Model file for the job. Use its own axes, mm. Face numbers are marked on the shaded views. A direction names the side the tool comes from. Coordinates: 2 decimals unless noted, no trailing zeros. Order: outer loops, then holes, each group sorted by start corner. A loop starts at its lowest first (then second) coordinate and runs counter-clockwise, first axis right, second up. Notation, with made-up numbers: M -1,33.25 L 27,33.25 A27 ccw 27,65.25 Z; hole C 23,65.5 d5. An arc over 180 degrees is marked long. Return JSON: item names as keys, results as strings.
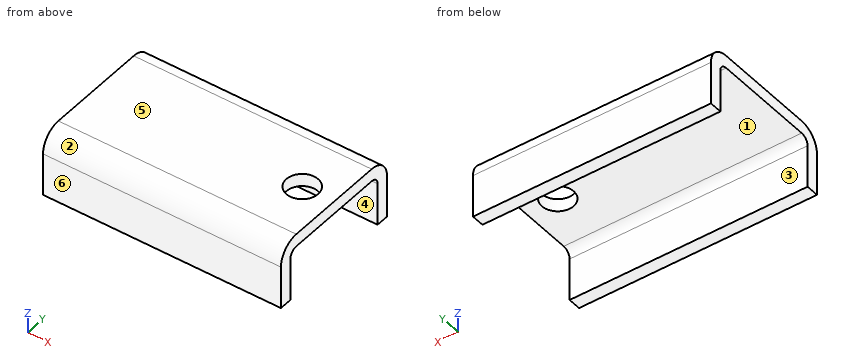
Autodesk Inventor part; units mm, degrees
ref_plane "YZ Plane" through (0, 0, 0) normal (1, 0, 0) x (0, 1, 0)
ref_plane "XZ Plane" through (0, 0, 0) normal (0, 1, 0) x (-1, 0, 0)
ref_plane "XY Plane" through (0, 0, 0) normal (0, 0, 1) x (1, 0, 0)
sketch "Sketch1" plane through (0, 0, 0) normal (0, 0, 1) x (1, 0, 0)
  line L0 (-75, -45) -> (75, -45)
  line L1 (75, -45) -> (75, 45)
  line L2 (75, 45) -> (-75, 45)
  line L3 (-75, 45) -> (-75, -45)
  line L4 (-75, -45) -> (75, 45) construction
  line L5 (75, -45) -> (-75, 45) construction
  circle A0 centre (55, -25) radius 10
  circle A1 centre (55, 25) radius 10
  line L6 (0, 0) -> (75, 0) construction
  circle A2 centre (55, 0) radius 10
  dimension "d0" = 150
  dimension "d1" = 90
  dimension "d23" = 20
  dimension "d25" = 20
  dimension "d26" = 20
extrude "Plate1" add sketch "Sketch1" along normal blind 8 contours L3 L2 L1 L0 | A0 | A1
sketch "Sketch6" plane through (-75, -37, 8) normal (0, -1, 0) x (1, 0, 0)
  line L0 (150, 0) -> (0, 0)
  line L1 (0, 0) -> (0, -40)
  line L2 (0, -40) -> (150, -40)
  line L3 (150, -40) -> (150, 0)
edge flange "Flange2" height 40 angle 90 thickness 8 bend radius 5 thickness toward (0, -1, 0) relief round relief width 8 relief depth 4 corner gap 5 corner form 0 edges at (0, -45, 0) (0, 45, 0) wall of the first edge with corners at (75, -37, 8) (-75, -37, 8) (-75, -37, -32) (75, -37, -32)
bend "Bend2"
corner "Corner2"
equation "\"d26\" = d25"
equation "\"d2\" = Thickness"
equation "\"d30\" = BendReliefWidth"
equation "\"d31\" = BendReliefDepth"
equation "\"d32\" = MinimumRemnant"
equation "\"d33\" = TransitionRadius"
equation "\"d36\" = BendRadius"
equation "\"d37\" = CornerReliefSize"
equation "\"d38\" = GapSize"
equation "\"d39\" = JacobiRadiusSize"
equation "\"BendReliefWidth\" = Thickness"
equation "\"BendReliefDepth\" = 0.5 * Thickness"
equation "\"CornerReliefSize\" = 4 * Thickness"
equation "\"MinimumRemnant\" = 2 * Thickness"
equation "\"TransitionRadius\" = BendRadius"
equation "\"JacobiRadiusSize\" = BendRadius"
equation "\"GapSize\" = Thickness"
properties part number "PNS 1785 leg floor channel_1200" material "Steel"
Item 1: Saw through at A-A (z = -20). Write the cut outline in (x, y).
Check result:
{"outline": "M -75,-45 L 75,-45 L 75,-37 L -75,-37 Z; M -75,37 L 75,37 L 75,45 L -75,45 Z"}
Item 2: Saw through at C-C (y = 0). Write the cut outline in (x, z).
Check result:
{"outline": "M -75,0 L 45,0 L 45,8 L -75,8 Z; M 65,0 L 75,0 L 75,8 L 65,8 Z"}
Item 3: Saw through at B-B (x = 55). Write the cut outline in (y, z).
Check result:
{"outline": "M -45,-32 L -37,-32 L -37,-5 A5 cw -32,0 L -10,0 L -10,8 L -32,8 A13 ccw -45,-5 Z; M 10,0 L 32,0 A5 cw 37,-5 L 37,-32 L 45,-32 L 45,-5 A13 ccw 32,8 L 10,8 Z"}
Item 4: Wall check: line 1 (Y direction, x = 30, z = -29.5); line 2 (Z direction, x = 52, y = 18.5); line 3 (Y direction, x = 55, z = 2). Give the ranges that are in metal, low to high.
Check result:
{"line 1": "y = -45 to -37, 37 to 45", "line 2": "z = 0 to 8", "line 3": "y = -42.95 to -10, 10 to 42.95"}
Item 5: Pull direction Y, two halves, no side cores. Call the marked faces 3, 4, 5 and 6: +Y half, -Y half, draft (parallel to the pull), parting line (faces both ways), or undercut.
Check result:
{"face 3": "undercut", "face 4": "undercut", "face 5": "draft", "face 6": "-Y half"}
Item 6: 3-axis set-ups, long thin cutter, end or side, ignore diameter. For the marked faces 1 and 2: which of +Z, -Z, +X, -X, +Y, -Y reach the whole face in a straight line?
Check result:
{"face 1": "-Z, +X, -X", "face 2": "+Z, +X, -X, -Y"}
Item 7: Drop flat-ended pins along their axis: pin 1 Ø16 at (x, y) = (55, 0) entering from +Z; pin 2 Ø2 at (x, y) = (-32, 21) entering from -Z. Give the stop position or say it passes through.
Check result:
{"pin 1": "passes through", "pin 2": "stops at z = 0"}
Item 8: Saw through at D-D (x = -1). Write the cut outline in (y, z), and give its area (3 significant figures).
Check result:
{"outline": "M -45,-32 L -37,-32 L -37,-5 A5 cw -32,0 L 32,0 A5 cw 37,-5 L 37,-32 L 45,-32 L 45,-5 A13 ccw 32,8 L -32,8 A13 ccw -45,-5 Z", "area": "1,170 mm2"}
